from build123d import *

# Parameters (mm, degrees)
SKETCH2_W                        = 150
SKETCH2_H                        = 90
SKETCH2_H_2                      = 60
BOSS_EXTRUDE1_DEPTH              = 15
SKETCH3_R                        = 13.005
SKETCH3_R_2                      = 3.01
CUT_EXTRUDE1_DEPTH               = 16
TAP_DRILL_FOR_M8X1_25_TAP1_D     = 6.8
TAP_DRILL_FOR_M8X1_25_TAP1_DEPTH = 10
TAP_DRILL_FOR_M8X1_25_TAP1_TIP   = 2.042926105


with BuildPart() as part:
    # Sketch2 → Boss-Extrude1 (new body)
    with BuildSketch(Plane.XY):
        Rectangle(SKETCH2_W, SKETCH2_H)
        with Locations((0, -75)):
            Rectangle(SKETCH2_W, SKETCH2_H_2)
        with BuildLine():
            Line((-75, -105), (75, -105))
            ThreePointArc((75, -105), (0, -136.066017178), (-75, -105))
        make_face()
    extrude(amount=BOSS_EXTRUDE1_DEPTH)

    # Sketch3 → Cut-Extrude1 (cut, through all)
    with BuildSketch(Plane.XY.offset(15)):
        with Locations((0, -85)):
            Circle(SKETCH3_R)
        with Locations((-29.444863729, -102)):
            Circle(SKETCH3_R_2)
        with Locations((0, -119)):
            Circle(SKETCH3_R_2)
    extrude(amount=-CUT_EXTRUDE1_DEPTH, mode=Mode.SUBTRACT)

    # Tap Drill for M8x1.25 Tap1
    with Locations(Plane(origin=(0, 0, 0), x_dir=(-1, 0, 0), z_dir=(0, 0, -1))):
        with Locations((-37.5, -50), (37.5, -50)):
            Hole(TAP_DRILL_FOR_M8X1_25_TAP1_D / 2, depth=TAP_DRILL_FOR_M8X1_25_TAP1_DEPTH)
            with Locations((0, 0, -(TAP_DRILL_FOR_M8X1_25_TAP1_DEPTH + TAP_DRILL_FOR_M8X1_25_TAP1_TIP / 2))):  # 118° drill point
                Cone(0, TAP_DRILL_FOR_M8X1_25_TAP1_D / 2, TAP_DRILL_FOR_M8X1_25_TAP1_TIP, mode=Mode.SUBTRACT)


solid = part.part
Input: part model. Units: mm. Frame: model coordinates. A direction names the side the tool comes from. Give positions to 0.01 mm unless a question says otherwise; leave off trailing zeros. Loops run counter-clockwise (first coordinate to the right, second up) from the corner with the lowest first, then second, coordinate; pieces in that order, holes last. Notation, with made-up numbers: (-2.75, 83) -> (23.25, 83) arc R37 ccw to (23.25, 121) -> close; hole circle Ø11 at (-20.5, 81.5). An arc over 180 degrees is marked (long way). Answer as a JSON object with one key per item and string values. Group by question number.
Item 1: Reachability of faces 1 (the cylindrical face through (39.328, -47.133, 5.07)), 2 (the flat face through (-1, 45, 7)) from +Z, -Z, +X, -X, +Y, -Y: full face, straight path, thin tool, end or side. Return the list, or none.
Item 2: Cut plane A-A, the plane x = 0. Return the cut outline in (y, z) (3 decimals), and give its area (3 significant figures).
Item 3: Cut plane D-D, the plane y = -78. Return the cut outline in (x, z).
Item 4: Cut plane C-C, the plane z = 3.5. Return the cut outline in (x, y) (3 decimals), and give its area (3 significant figures).
Item 5: Pull-direction query (Y, two-part tool) for faces 3 (the cylindrical face through (-0.65, -121.94, 7.6)), 4 (the flat face through (-1, -44, 0)), 5 (the cylindrical face through (1.17, -136.06, 7.4)); classes: released by +Y, released by -Y, zero draft, split by the parting line, or undercut.
Item 6: Line query: probe 1 along Y at (x, z) = (0, 8.75) (3 decimals); probe 2 along X at (y, z) = (-50, 5.5); probe 3 along X at (y, z) = (-84.5, 3.75). Output: solid intervals per line, ascending.
Item 7: Cut plane B-B, the plane y = -102. Return the cut outline in (x, z).
Item 8: Pin query (flat end, axial travel): P1, Ø3, axis at y = -113, z = 7.5, coming from the -X side; P2, Ø1, axis at x = -31, z = 3.5, coming from the -Y side; P3, Ø3, axis at x = 10, z = 3, coming from the -Y side. Return the tip coordinate at first contact, or that it passes through.
Checks:
{
 "1": {"face 1": "-Z", "face 2": "+Z, -Z, +X, -X, +Y"},
 "2": {"outline": "(-136.066, 0) -> (-122.01, 0) -> (-122.01, 15) -> (-136.066, 15) -> close; (-115.99, 0) -> (-98.005, 0) -> (-98.005, 15) -> (-115.99, 15) -> close; (-71.995, 0) -> (45, 0) -> (45, 15) -> (-71.995, 15) -> close", "area": "2,240 mm²"},
 "3": {"outline": "(-75, 0) -> (-10.96, 0) -> (-10.96, 15) -> (-75, 15) -> close; (10.96, 0) -> (75, 0) -> (75, 15) -> (10.96, 15) -> close"},
 "4": {"outline": "(-75, -105) arc R106.066 ccw to (75, -105) -> (75, 45) -> (-75, 45) -> close; hole circle Ø6.8 at (-37.5, -50); hole circle Ø6.02 at (-29.445, -102); hole circle Ø26.01 at (0, -85); hole circle Ø6.02 at (0, -119); hole circle Ø6.8 at (37.5, -50)", "area": "25,000 mm²"},
 "5": {"face 3": "undercut", "face 4": "zero draft", "face 5": "released by -Y"},
 "6": {"probe 1": "y = -136.066 to -122.01, -115.99 to -98.005, -71.995 to 45", "probe 2": "x = -75 to -40.9, -34.1 to 34.1, 40.9 to 75", "probe 3": "x = -75 to -13, 13 to 75"},
 "7": {"outline": "(-75, 0) -> (-32.45, 0) -> (-32.45, 15) -> (-75, 15) -> close; (-26.43, 0) -> (75, 0) -> (75, 15) -> (-26.43, 15) -> close"},
 "8": {"P1": "stops at x = -67.88", "P2": "stops at y = -131.59", "P3": "stops at y = -135.72"}
}
